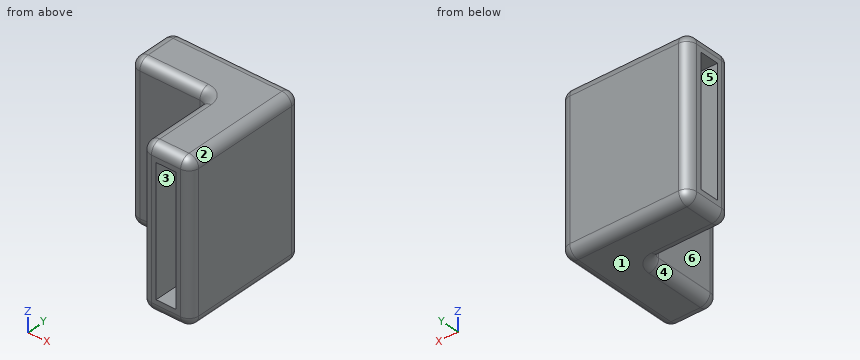
```python
from build123d import *

# Parameters (mm, degrees)
F0_W     = 35
F0_H     = 10.1
F0_W_2   = 10.1
F0_H_2   = 35
F1_DEPTH = 80
F3_W     = 10.1
F3_H     = 65.1
F4_DEPTH = 35
F2_W     = 10.1
F2_H     = 65.1
F5_DEPTH = 35
F6_R     = 5


with BuildPart() as f1:
    # F0 (on Top) → F1 (new body)
    with BuildSketch(Plane.XY):
        with BuildLine():
            Line((0, 7.45), (0, 0))
            Line((0, 0), (35.8354191061, 0))
            ThreePointArc((35.8354191061, 0), (39.370953012, -1.4644660941), (40.8354191061, -5))
            Line((40.8354191061, -5), (40.8354191061, -40.8354191061))
            Line((40.8354191061, -40.8354191061), (48.2854191061, -40.8354191061))
            Line((48.2854191061, -40.8354191061), (48.2854191061, -5.8354191061))
            Line((48.2854191061, -5.8354191061), (58.3854191061, -5.8354191061))
            Line((58.3854191061, -5.8354191061), (58.3854191061, -40.8354191061))
            Line((58.3854191061, -40.8354191061), (65.8354191061, -40.8354191061))
            Line((65.8354191061, -40.8354191061), (65.8354191061, 20))
            ThreePointArc((65.8354191061, 20), (64.370953012, 23.5355339059), (60.8354191061, 25))
            Line((60.8354191061, 25), (0, 25))
            Line((0, 25), (0, 17.55))
            Line((0, 17.55), (35, 17.55))
            Line((35, 17.55), (35, 7.45))
            Line((35, 7.45), (0, 7.45))
        make_face()
        with Locations((17.5, 12.5)):
            Rectangle(F0_W, F0_H)
        with Locations((53.3354191061, -23.3354191061)):
            Rectangle(F0_W_2, F0_H_2)
    extrude(amount=F1_DEPTH)

    # F3 (on face) → F4 (cut)
    with BuildSketch(Plane.XZ.offset(40.8354191061)):
        with Locations((53.3354191061, 40)):
            Rectangle(F3_W, F3_H)
    extrude(amount=-F4_DEPTH, mode=Mode.SUBTRACT)

    # F2 (on face) → F5 (cut)
    with BuildSketch(Plane(origin=(0, 0, 0), x_dir=(0, -1, 0), z_dir=(-1, 0, 0))):
        with Locations((-12.5, 40)):
            Rectangle(F2_W, F2_H)
    extrude(amount=-F5_DEPTH, mode=Mode.SUBTRACT)

    # F6
    f6_edges = [f1.edges().sort_by_distance(p)[0] for p in [
        (64.370953, 23.535534, 80),
        (30.41771, 25, 80),
        (0, 12.5, 80),
        (17.91771, 0, 80),
        (39.370953, -1.464466, 80),
        (40.835419, -22.91771, 80),
        (53.335419, -40.835419, 80),
        (65.835419, -10.41771, 80),
        (64.370953, 23.535534, 0),
        (30.41771, 25, 0),
        (0, 12.5, 0),
        (17.91771, 0, 0),
        (39.370953, -1.464466, 0),
        (40.835419, -22.91771, 0),
        (53.335419, -40.835419, 0),
        (65.835419, -10.41771, 0),
        (65.835419, -40.835419, 40),
        (40.835419, -40.835419, 40),
        (0, 0, 40),
        (0, 25, 40),
    ]]
    fillet(f6_edges, radius=F6_R)


solid = f1.part
```
Here's how the part is built. I have some questions about the finished solid (model axes, mm). Face numbers are marked on the shaded views. A direction names the side the tool comes from. Give positions to 0.01 mm unless a question says otherwise; leave off trailing zeros. Write each loop counter-clockwise with the first axis right and the second up, starting at its lowest first coordinate (ties: lowest second). Pieces come first, ordered by that corner, then holes. Notation, with made-up numbers: M -40,-19 L 1,-19 A19 ccw 1,11 Z; hole C 78.25,-15 d11. An arc over 180 degrees is marked long. Put each result on its own line as item: value. Start each with the question number.
Item 1: On a 3-axis mill with a long thin cutter (end or side, diameter ignored), from which of +Z, -Z, +X, -X, +Y, -Y can I reach the whole of each face in a straight line? I mean the marked faces 4, 5 and 6. Say none if no direction works.
Item 2: If we section it at A-A, the plane y = -29.5: Write out the boundary of the cut face in (x, z), then the cut area to 3 significant figures.
Item 3: If we section it at B-B, the plane z = 69: Write out the boundary of the cut face in (x, y), then the cut area to 3 significant figures.
Item 4: Will these pins go through, and if not, where does the flat tip stop? pin 1 (9.5 mm diameter, centred on x = 27.5, z = 48, fed in from -Y); pin 2 (9.5 mm diameter, centred on y = -14.5, z = 30, fed in from -X); pin 3 (1.5 mm diameter, centred on x = 55.5, z = 40.5, fed in from -Y).
Item 5: Thinking about a two-plate mould opening in X: for the marked faces 1, 2 and 3, which applies, +X half, -X half, draft (parallel to the pull), parting line (faces both ways), or undercut?
Item 6: If we section it at D-D, the plane y = 14.5: Write out the boundary of the cut face in (x, z).
Item 7: If we section it at C-C, the plane x = 22: Write out the boundary of the cut face in (y, z), then the cut area to 3 significant figures.
Item 8: I need wall thicknesses on L1, parallel to Y at x = 28, z = 12.5; L2, parallel to X at y = -33, z = 58; L3, parallel to Z at x = 52.5, y = -13. Which ranges of each line are inside material? Lowest first, please. Write a range as from..to.
Values:
1. face 4: -Z, -X, -Y
1. face 5: -X
1. face 6: +Z, -Z, -X, -Y
2. outline: M 40.84,5 A5 ccw 45.84,0 L 60.84,0 A5 ccw 65.84,5 L 65.84,75 A5 ccw 60.84,80 L 45.84,80 A5 ccw 40.84,75 Z; hole M 48.29,7.45 L 58.39,7.45 L 58.39,72.55 L 48.29,72.55 Z
2. area: 1,320 mm²
3. outline: M 0,5 A5 ccw 5,0 L 35.84,0 A5 cw 40.84,-5 L 40.84,-35.84 A5 ccw 45.84,-40.84 L 48.29,-40.84 L 48.29,-5.84 L 58.39,-5.84 L 58.39,-40.84 L 60.84,-40.84 A5 ccw 65.84,-35.84 L 65.84,20 A5 ccw 60.84,25 L 5,25 A5 ccw 0,20 L 0,17.55 L 35,17.55 L 35,7.45 L 0,7.45 Z
3. area: 1,940 mm²
4. pin 1: y = 0
4. pin 2: x = 40.84
4. pin 3: y = -5.84
5. face 1: draft
5. face 2: +X half
5. face 3: undercut
6. outline: M 0,5 A5 ccw 5,0 L 60.84,0 A5 ccw 65.84,5 L 65.84,75 A5 ccw 60.84,80 L 5,80 A5 ccw 0,75 L 0,72.55 L 35,72.55 L 35,7.45 L 0,7.45 Z
7. outline: M 0,5 A5 ccw 5,0 L 20,0 A5 ccw 25,5 L 25,75 A5 ccw 20,80 L 5,80 A5 ccw 0,75 Z; hole M 7.45,7.45 L 17.55,7.45 L 17.55,72.55 L 7.45,72.55 Z
7. area: 1,320 mm²
8. L1: 0..7.45, 17.55..25
8. L2: 40.84..48.29, 58.39..65.84
8. L3: 0..7.45, 72.55..80
